```python
from build123d import *

# Parameters (mm, degrees)
ESQUISSE1_R        = 1.61
BOSS_EXTRU_1_DEPTH = 1.5


with BuildPart() as part:
    # Esquisse1 → Boss.-Extru.1 (new body)
    with BuildSketch(Plane.XY):
        with BuildLine():
            Line((31.265, 25.65), (31.265, 14.15))
            Line((31.265, 14.15), (34.265, 11.15))
            Line((34.265, 11.15), (34.265, -20.85))
            Line((34.265, -20.85), (31.265, -23.85))
            Line((31.265, -23.85), (31.265, -25.65))
            ThreePointArc((31.265, -25.65), (30.972106781, -26.357106781), (30.265, -26.65))
            Line((30.265, -26.65), (-33.265, -26.65))
            ThreePointArc((-33.265, -26.65), (-33.972106781, -26.357106781), (-34.265, -25.65))
            Line((-34.265, -25.65), (-34.265, 25.65))
            ThreePointArc((-34.265, 25.65), (-33.972106781, 26.357106781), (-33.265, 26.65))
            Line((-33.265, 26.65), (30.265, 26.65))
            ThreePointArc((30.265, 26.65), (30.972106781, 26.357106781), (31.265, 25.65))
        make_face()
        with Locations((32.265, 8.92)):
            Circle(ESQUISSE1_R, mode=Mode.SUBTRACT)
        with Locations((32.265, -18.98)):
            Circle(ESQUISSE1_R, mode=Mode.SUBTRACT)
        with Locations((-18.495, 24.15)):
            Circle(ESQUISSE1_R, mode=Mode.SUBTRACT)
    extrude(amount=BOSS_EXTRU_1_DEPTH)


solid = part.part
```
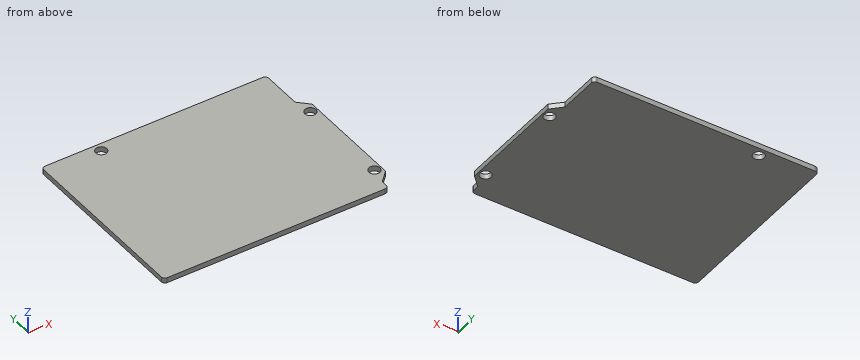
The model under review builds one solid part; all positions refer to its coordinate system, in mm. Round coordinates to 2 decimals unless told otherwise and drop trailing zeros. Write each loop counter-clockwise with the first axis right and the second up, starting at its lowest first coordinate (ties: lowest second). Pieces come first, ordered by that corner, then holes. Notation, with made-up numbers: M -37.75,7 L -22.75,7 A30 ccw -22.75,36 Z; hole C -33.75,37.5 d11. An arc over 180 degrees is marked long. Use CSV: the item, a comma, the result in double quotes. Start each with the question number.
(1) We need section B-B, the plane z = 1.05. State the section outline as (x, y) points (3 decimals), then the cut area to 3 significant figures.
(2) For line 1 along X through (y, z) = (22.5, 1.3) (3 decimals); line 2 along X through (y, z) = (23, 0.15) (3 decimals), list the stretches that pass through material, from the lowest coordinate up.
(3) Clearance check with a flat-ended pin moving along its axis: P1, Ø1.9, axis at x = 32.265, y = -18.98, coming from the +Z side. State where the tip first meets the part, or that it passes through.
(4) We need section C-C, the plane y = -18.98. State the section outline as (x, z) points (3 decimals).
(5) We need section A-A, the plane y = 24.15. State the section outline as (x, z) points (3 decimals), then the cut area to 3 significant figures.
Findings:
1,outline,"M -34.265,-25.65 A1 ccw -33.265,-26.65 L 30.265,-26.65 A1 ccw 31.265,-25.65 L 31.265,-23.85 L 34.265,-20.85 L 34.265,11.15 L 31.265,14.15 L 31.265,25.65 A1 ccw 30.265,26.65 L -33.265,26.65 A1 ccw -34.265,25.65 Z; hole C -18.495,24.15 d3.22; hole C 32.265,-18.98 d3.22; hole C 32.265,8.92 d3.22"
1,area,"3,570 mm^2"
2,line 1,"-34.265 to 31.265"
2,line 2,"-34.265 to -19.622, -17.368 to 31.265"
3,P1,"through"
4,outline,"M -34.265,0 L 30.655,0 L 30.655,1.5 L -34.265,1.5 Z; M 33.875,0 L 34.265,0 L 34.265,1.5 L 33.875,1.5 Z"
5,outline,"M -34.265,0 L -20.105,0 L -20.105,1.5 L -34.265,1.5 Z; M -16.885,0 L 31.265,0 L 31.265,1.5 L -16.885,1.5 Z"
5,area,"93.5 mm^2"
